The drawing under review shows one solid part. Ordinate dimensions are in mm from its lowest x, y, z. Coordinates: 2 decimals unless noted, no trailing zeros. Write each loop counter-clockwise with the first axis right and the second up, starting at its lowest first coordinate (ties: lowest second). Pieces come first, ordered by that corner, then holes. Notation, with made-up numbers: M 47.5,-25.75 L 92.5,-25.75 A23 ccw 92.5,-2.75 Z; hole C 89.25,20.25 d7. An arc over 180 degrees is marked long. Write each question's results on one line, items separated by ' | '. Start each with the question number.
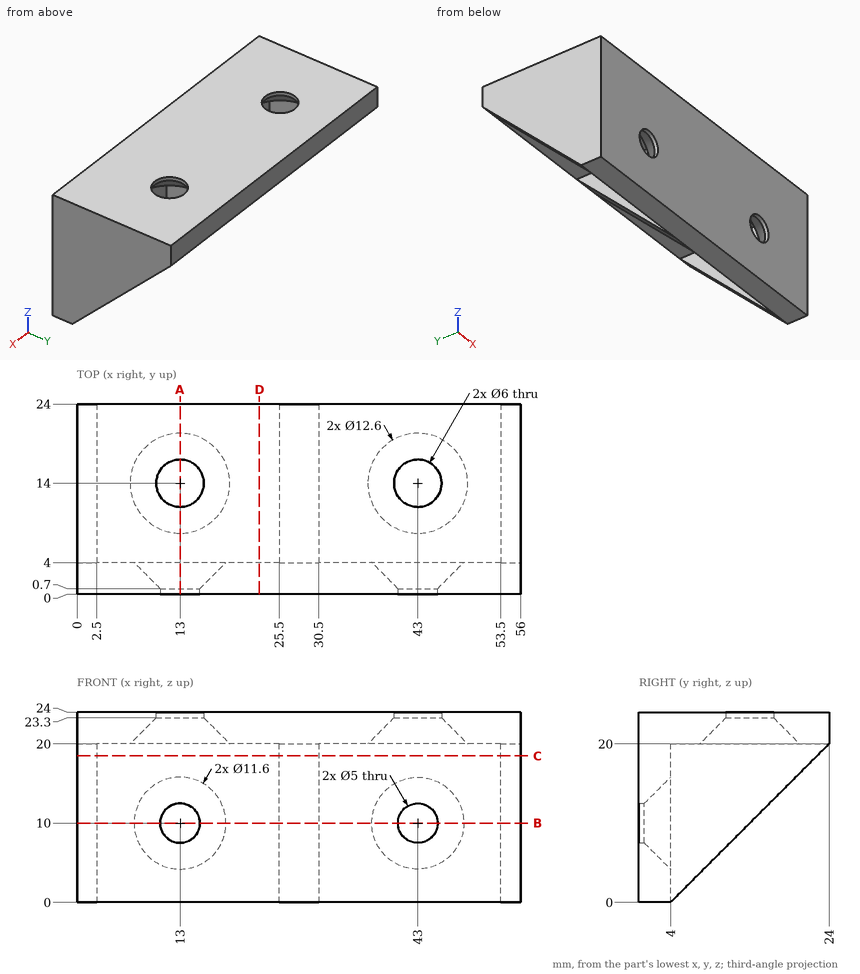
Item 1: We need section B-B on z = 10. State the section outline as (x, y) points.
Item 2: We need section C-C on z = 18.5. State the section outline as (x, y) points.
Item 3: We need section A-A on x = 13. State the section outline as (y, z) points, then the cut area to 3 significant figures.
Item 4: We need section D-D on x = 23. State the section outline as (y, z) points, then the cut area to 3 significant figures.
Item 5: Wall thickness on L1, parallel to X at y = 14, z = 23.85; L2, parallel to X at y = 10.75, z = 8; L3, parallel to Y at x = 43, z = 23.6: over which ranges is each line inside the solid? List them lowest first.
Item 6: Insertion check: pin 1 Ø4 at (x, z) = (13, 10) entering from -Y; pin 2 Ø8 at (x, z) = (43, 10) entering from +Y; pin 3 Ø1.5 at (x, z) = (16.5, 16.5) entering from +Y; pin 4 Ø4 at (x, y) = (22, 12) entering from -Z. Each pin has a flat end and moves straight along its axis. Give the tip position at first contact, or say it passes through.
Answer:
1) outline: M 0,0 L 10.5,0 L 10.5,0.7 L 7.2,4 L 2.5,4 L 2.5,14 L 0,14 Z; M 15.5,0 L 40.5,0 L 40.5,0.7 L 37.2,4 L 30.5,4 L 30.5,14 L 25.5,14 L 25.5,4 L 18.8,4 L 15.5,0.7 Z; M 45.5,0 L 56,0 L 56,14 L 53.5,14 L 53.5,4 L 48.8,4 L 45.5,0.7 Z
2) outline: M 0,0 L 56,0 L 56,22.5 L 53.5,22.5 L 53.5,4 L 30.5,4 L 30.5,22.5 L 25.5,22.5 L 25.5,4 L 2.5,4 L 2.5,22.5 L 0,22.5 Z
3) outline: M 0,0 L 4,0 L 4,4.2 L 0.7,7.5 L 0,7.5 Z; M 0,12.5 L 0.7,12.5 L 4,15.8 L 4,20 L 7.7,20 L 11,23.3 L 11,24 L 0,24 Z; M 17,23.3 L 20.3,20 L 24,20 L 24,24 L 17,24 Z | area: 110 mm^2
4) outline: M 0,0 L 4,0 L 4,20 L 24,20 L 24,24 L 0,24 Z | area: 176 mm^2
5) L1: x = 0 to 10, 16 to 40, 46 to 56 | L2: x = 0 to 2.5, 25.5 to 30.5, 53.5 to 56 | L3: y = 0 to 11, 17 to 24
6) pin 1: passes through | pin 2: stops at y = 2.2 | pin 3: stops at y = 4 | pin 4: stops at z = 20
